Read the model definition and answer for the solid it produces. Units are mm, in the model's axes. Face numbers are marked on the shaded views. A direction names the side the tool comes from. Coordinates: 2 decimals unless noted, no trailing zeros. Loops run counter-clockwise (first coordinate to the right, second up) from the corner with the lowest first, then second, coordinate; pieces in that order, holes last. Notation, with made-up numbers: (6.25, 25) - (64.25, 25) arc R32 ccw to (64.25, 56) - close; hole circle Ø7 at (83, -4). An arc over 180 degrees is marked (long way). Use one line per item in the form item = value. Start each with the question number.
1) Which of the six approach directions +Z, -Z, +X, -X, +Y, -Y give full straight-line access (tool end or side, diameter ignored) to the marked faces 1 and 2?
2) A cutting plane is placed at D-D (z = 66.31). Give the vertices of the cut face in (x, y).
3) Each of these flat-tipped pins is pushed along its axis until it touches: P1, Ø7, axis at x = 1, y = 0, coming from the +Z side; P2, Ø12, axis at y = 23, z = 58, coming from the +X side. Where does it stop, or does it pass through?
4) A cutting plane is placed at A-A (x = -9.5). Give the vertices of the cut face in (y, z).
5) A cutting plane is placed at C-C (x = 1). Give the vertices of the cut face in (y, z).
6) Consider line 1 (Y direction, x = 1, z = 1); line 2 (Y direction, x = -36.55, z = 19.21); line 3 (Y direction, x = -37.1, z = 42.76). Determine where each line is inside the solid, lowest interval first.
7) A cutting plane is placed at B-B (y = 0). Give the vertices of the cut face in (x, z).
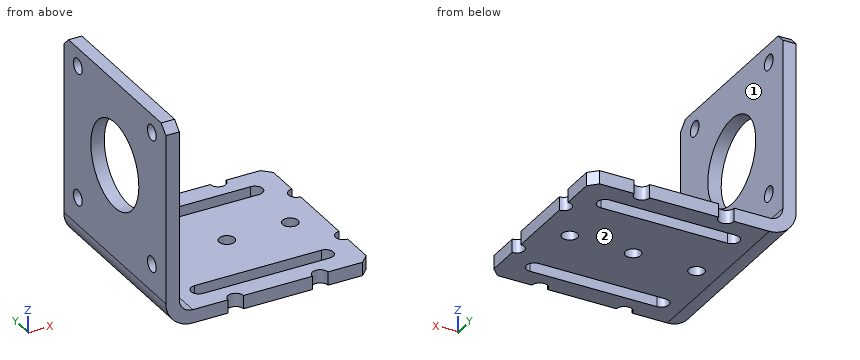
Autodesk Inventor part; units mm, degrees
ref_plane "YZ Plane" through (0, 0, 0) normal (1, 0, 0) x (0, 1, 0)
ref_plane "XZ Plane" through (0, 0, 0) normal (0, 1, 0) x (-1, 0, 0)
ref_plane "XY Plane" through (0, 0, 0) normal (0, 0, 1) x (1, 0, 0)
sketch "Sketch1" plane through (0, 0, 0) normal (0, 0, 1) x (1, 0, 0)
  line L0 (-34, -32.5) -> (34, -32.5)
  line L1 (34, -32.5) -> (34, 32.5)
  line L2 (34, 32.5) -> (-34, 32.5)
  line L3 (-34, 32.5) -> (-34, -32.5)
  line L4 (-34, -32.5) -> (34, 32.5) construction
  line L5 (34, -32.5) -> (-34, 32.5) construction
  point P0 (0, 0)
  dimension "d0" = 68
  dimension "d1" = 65
extrude "Plate1" add sketch "Sketch1" along normal blind 4.76
sketch "Sketch2" plane through (-34, -32.5, 4.76) normal (-1, 0, 0) x (0, -1, 0)
  line L0 (-65, 0) -> (0, 0)
  line L1 (0, 0) -> (0, 68)
  line L2 (0, 68) -> (-65, 68)
  line L3 (-65, 68) -> (-65, 0)
edge flange "Flange1" height 72.76 angle 90 thickness 4.76 bend radius 4.76 thickness toward (-1, 0, 0) relief tear relief width 4.76 relief depth 2.38 edges at (-34, 0, 4.76) wall of the first edge with corners at (-34, 32.5, 4.76) (-34, -32.5, 4.76) (-34, -32.5, 72.76) (-34, 32.5, 72.76)
bend "Bend1"
corner "Corner1"
sketch "Sketch3" plane through (0, 0, 4.76) normal (0, 0, 1) x (1, 0, 0)
  line L0 (-29.24, 32.5) -> (-29.24, -32.5) construction
  line L1 (34, -32.5) -> (-29.24, -32.5) construction
  line L2 (34, 32.5) -> (34, -32.5) construction
  line L3 (-29.24, 32.5) -> (34, 32.5) construction
  line L4 (-29.24, 32.5) -> (34, 32.5)
  circle A0 centre (-14, 32.5) radius 2.75
  circle A1 centre (16, 32.5) radius 2.75
  line L5 (34, 32.5) -> (34, -32.5) construction
  line L6 (34, 0) -> (-29.24, 0) construction
  line L7 (-29.24, 32.5) -> (-29.24, -32.5) construction
  arc A2 (-21.5, 25.25) -> (-21.5, 19.75) centre (-21.5, 22.5) ccw
  arc A3 (20.75, 22.5) -> (23.5, 19.75) centre (23.5, 22.5) ccw construction
  line L8 (-21.5, 22.5) -> (23.5, 22.5) construction
  line L9 (-21.5, 25.25) -> (23.5, 25.25)
  line L10 (23.5, 19.75) -> (-21.5, 19.75)
  arc A4 (-18.75, 22.5) -> (-21.5, 25.25) centre (-21.5, 22.5) ccw construction
  arc A5 (-21.5, 19.75) -> (-18.75, 22.5) centre (-21.5, 22.5) ccw construction
  arc A6 (23.5, 25.25) -> (20.75, 22.5) centre (23.5, 22.5) ccw construction
  arc A7 (23.5, 19.75) -> (23.5, 25.25) centre (23.5, 22.5) ccw
  circle A8 centre (34, 15) radius 2.75
  circle A9 centre (-14, -32.5) radius 2.75
  circle A10 centre (16, -32.5) radius 2.75
  arc A11 (-21.5, -19.75) -> (-21.5, -25.25) centre (-21.5, -22.5) ccw
  line L11 (-21.5, -25.25) -> (23.5, -25.25)
  line L12 (23.5, -19.75) -> (-21.5, -19.75)
  arc A12 (23.5, -25.25) -> (23.5, -19.75) centre (23.5, -22.5) ccw
  circle A13 centre (34, -15) radius 2.75
  line L13 (-21.5, 22.5) -> (-21.5, -22.5) construction
  line L14 (23.5, 22.5) -> (23.5, -22.5) construction
  line L15 (23.5, -22.5) -> (-21.5, -22.5) construction
  line L16 (1, -22.5) -> (1, 22.5) construction
  circle A14 centre (-21.5, 0) radius 2.75
  circle A15 centre (1, 0) radius 2.75
  circle A16 centre (23.5, 0) radius 2.75
  point P0 (0, 0)
  dimension "d13" = 5.5
  dimension "d14" = 30
  dimension "d15" = 18
  dimension "d16" = 5.5
  dimension "d17" = 45
  dimension "d18" = 10.5
  dimension "d19" = 45
  dimension "d20" = 30
extrude "Cut1" cut sketch "Sketch3" against normal blind 4.76
sketch "Sketch4" plane through (-34, -32.5, 72.76) normal (1, 0, 0) x (0, 0, -1)
  line L0 (63.24, 0) -> (63.24, 65) construction
  line L1 (0, 65) -> (63.24, 65) construction
  line L2 (0, 65) -> (0, 0) construction
  line L3 (0, 0) -> (63.24, 0) construction
  line L4 (0, 65) -> (0, 0) construction
  line L5 (0, 32.5) -> (63.24, 32.5) construction
  circle A0 centre (30, 32.5) radius 15.25
  line L6 (53.55, 8.95) -> (6.45, 8.95) construction
  line L7 (6.45, 8.95) -> (6.45, 56.05) construction
  line L8 (6.45, 56.05) -> (53.55, 56.05) construction
  line L9 (53.55, 56.05) -> (53.55, 8.95) construction
  line L10 (53.55, 8.95) -> (6.45, 56.05) construction
  line L11 (6.45, 8.95) -> (53.55, 56.05) construction
  circle A1 centre (6.45, 8.95) radius 2.75
  circle A2 centre (6.45, 56.05) radius 2.75
  circle A3 centre (53.55, 56.05) radius 2.75
  circle A4 centre (53.55, 8.95) radius 2.75
  point P0 (72.76, 32.5)
  dimension "d23" = 30
  dimension "d24" = 30.5
  dimension "d25" = 47.1
  dimension "d26" = 5.5
extrude "Cut2" cut sketch "Sketch4" against normal blind 4.76
chamfer "Corner Chamfer1" distance 3 angle 45 4 edges at (-36.38, 32.5, 72.76) (-36.38, -32.5, 72.76) (34, -32.5, 2.38) (34, 32.5, 2.38)
equation "\"d21\" = Thickness"
equation "\"d27\" = Thickness"
equation "\"d3\" = BendReliefWidth"
equation "\"d4\" = BendReliefDepth"
equation "\"d5\" = MinimumRemnant"
equation "\"d6\" = BendRadius"
equation "\"d9\" = BendRadius"
equation "\"d10\" = CornerReliefSize"
equation "\"d11\" = GapSize"
equation "\"d12\" = JacobiRadiusSize"
equation "\"BendRadius\" = Thickness"
equation "\"BendReliefWidth\" = Thickness"
equation "\"BendReliefDepth\" = 0.5 * Thickness"
equation "\"CornerReliefSize\" = 4 * Thickness"
equation "\"MinimumRemnant\" = 2 * Thickness"
equation "\"TransitionRadius\" = BendRadius"
equation "\"JacobiRadiusSize\" = BendRadius"
equation "\"GapSize\" = Thickness"
equation "\"d2\" = BendRadius"
properties part number "nema_support_techmakers" material "Steel, Alloy"
Found:
q1.face_1 = +Z, +X, +Y, -Y
q1.face_2 = -Z, +X, -X, +Y, -Y
q2.outline = (-38.76, -32.5) - (-34, -32.5) - (-34, -26.3) - (-38.76, -26.3) - close; (-38.76, -20.8) - (-34, -20.8) - (-34, 20.8) - (-38.76, 20.8) - close; (-38.76, 26.3) - (-34, 26.3) - (-34, 32.5) - (-38.76, 32.5) - close
q3.P1 = 4.76
q3.P2 = -34
q4.outline = (-32.5, 0) - (-25.25, 0) - (-25.25, 4.76) - (-32.5, 4.76) - close; (-19.75, 0) - (19.75, 0) - (19.75, 4.76) - (-19.75, 4.76) - close; (25.25, 0) - (32.5, 0) - (32.5, 4.76) - (25.25, 4.76) - close
q5.outline = (-32.5, 0) - (-25.25, 0) - (-25.25, 4.76) - (-32.5, 4.76) - close; (-19.75, 0) - (-2.75, 0) - (-2.75, 4.76) - (-19.75, 4.76) - close; (2.75, 0) - (19.75, 0) - (19.75, 4.76) - (2.75, 4.76) - close; (25.25, 0) - (32.5, 0) - (32.5, 4.76) - (25.25, 4.76) - close
q6.line_1 = -32.5 to -25.25, -19.75 to -2.75, 2.75 to 19.75, 25.25 to 32.5
q6.line_2 = -32.5 to -26.3, -20.8 to 20.8, 26.3 to 32.5
q6.line_3 = -32.5 to -15.25, 15.25 to 32.5
q7.outline = (-38.76, 9.52) arc R9.52 ccw to (-29.24, 0) - (-24.25, 0) - (-24.25, 4.76) - (-29.24, 4.76) arc R4.76 cw to (-34, 9.52) - (-34, 27.51) - (-38.76, 27.51) - close; (-38.76, 58.01) - (-34, 58.01) - (-34, 72.76) - (-38.76, 72.76) - close; (-18.75, 0) - (-1.75, 0) - (-1.75, 4.76) - (-18.75, 4.76) - close; (3.75, 0) - (20.75, 0) - (20.75, 4.76) - (3.75, 4.76) - close; (26.25, 0) - (34, 0) - (34, 4.76) - (26.25, 4.76) - close
